Verification items for this drawing (mm, ordinates from the low corner). Give positions to 0.01 mm unless a question says otherwise; leave off trailing zeros. Loops run counter-clockwise (first coordinate to the right, second up) from the corner with the lowest first, then second, coordinate; pieces in that order, holes last. Notation, with made-up numbers: (85, -38.5) -> (133, -38.5) arc R7 ccw to (133, -30.5) -> close; hole circle Ø3 at (-15, 54). An arc over 180 degrees is marked (long way). Answer as CSV lines item,"result". Start each with the question number.
(1) Section check A-A on y = 0.95. Enter the section's corners in (x, z).
(2) Section check C-C on x = 14.5. Enter the section's corners in (y, z), plus the area to 3 significant figures.
(3) Gauge pin test, flat end, axial feed: pin 1 Ø4 at (x, z) = (23, 28.5) entering from -Y. Record the tip position at first contact, or that the pin passes through.
(4) Material ranges on line 1 (X direction, y = 0.55, z = 19.5); line 2 (X direction, y = 1.65, z = 13); line 3 (Z direction, x = 35.5, y = 0.85), recorded low to high. Write a range as from..to.
(5) Section check B-B on z = 20. Enter the section's corners in (x, y), plus the area to 3 significant figures.
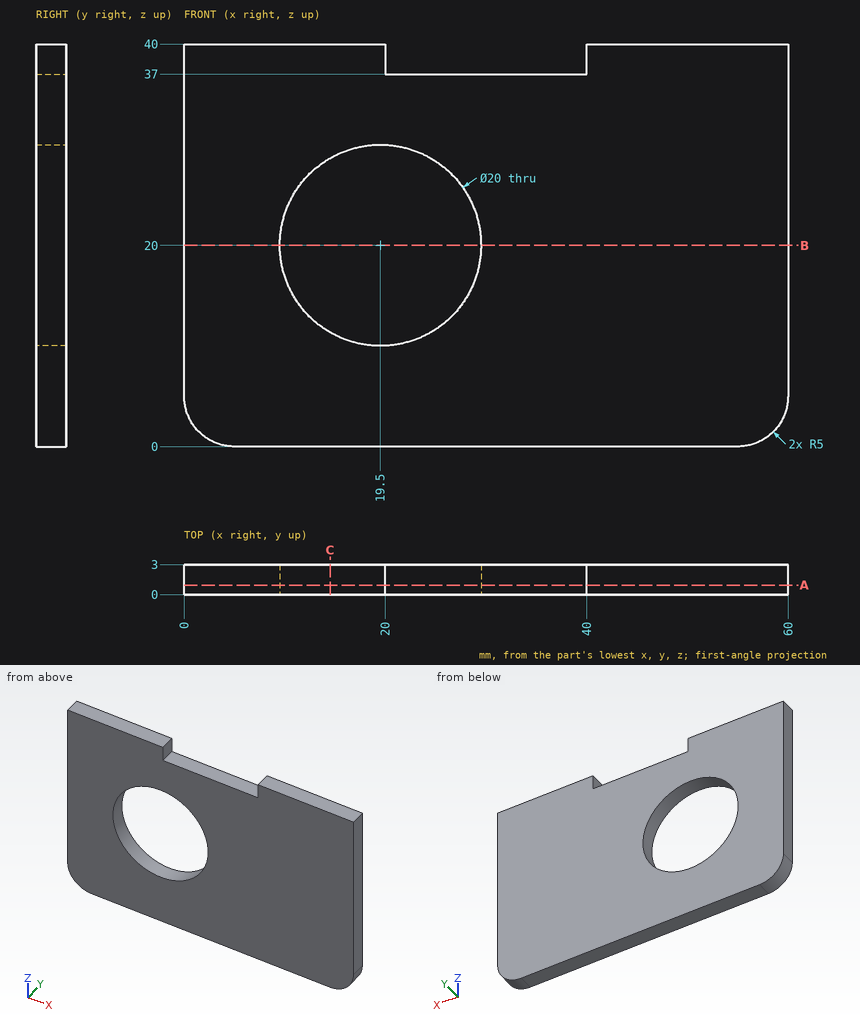
Working result:
1,outline,"(0, 5) arc R5 ccw to (5, 0) -> (55, 0) arc R5 ccw to (60, 5) -> (60, 40) -> (40, 40) -> (40, 37) -> (20, 37) -> (20, 40) -> (0, 40) -> close; hole circle Ø20 at (19.5, 20)"
2,outline,"(0, 0) -> (3, 0) -> (3, 11.34) -> (0, 11.34) -> close; (0, 28.66) -> (3, 28.66) -> (3, 40) -> (0, 40) -> close"
2,area,"68.0 mm^2"
3,pin 1,"stops at y = 0"
4,line 1,"x = 0..9.51, 29.49..60"
4,line 2,"x = 0..12.36, 26.64..60"
4,line 3,"z = 0..37"
5,outline,"(0, 0) -> (9.5, 0) -> (9.5, 3) -> (0, 3) -> close; (29.5, 0) -> (60, 0) -> (60, 3) -> (29.5, 3) -> close"
5,area,"120 mm^2"
